from build123d import *

# Parameters (mm, degrees)
SKETCH_1_W               = 764
SKETCH_1_H               = 732
EXTRUDE_1_DEPTH          = 18
SKETCH_1_3_W             = 28
SKETCH_1_3_H             = 60
EXTRUDE_2_DEPTH          = 18
PATTERN_LINEAR_1_COUNT   = 3
PATTERN_LINEAR_1_PITCH   = 250
MIRROR_1_COPY_1_SKETCH_W = 28
MIRROR_1_COPY_1_SKETCH_H = 60
MIRROR_1_COPY_1_DEPTH    = 18
MIRROR_1_COPY_2_SKETCH_W = 28
MIRROR_1_COPY_2_SKETCH_H = 60
MIRROR_1_COPY_2_DEPTH    = 18
SKETCH_1_5_W             = 60
SKETCH_1_5_H             = 28
EXTRUDE_3_DEPTH          = 18
PATTERN_LINEAR_2_COUNT   = 3
PATTERN_LINEAR_2_PITCH   = 250
MIRROR_2_COPY_1_SKETCH_W = 60
MIRROR_2_COPY_1_SKETCH_H = 28
MIRROR_2_COPY_1_DEPTH    = 18
MIRROR_2_COPY_2_SKETCH_W = 60
MIRROR_2_COPY_2_SKETCH_H = 28
MIRROR_2_COPY_2_DEPTH    = 18
FILLET_1_R               = 25


with BuildPart() as part:
    # 草图1 → 凸台-拉伸1 (new body)
    with BuildSketch(Plane(origin=(0, 0, 0), x_dir=(1, 0, 0), z_dir=(0, 1, 0))):
        Rectangle(SKETCH_1_W, SKETCH_1_H)
    extrude(amount=EXTRUDE_1_DEPTH)

    # 草图1<3> → 凸台-拉伸2 (add)
    with BuildSketch(Plane(origin=(0, 0, 0), x_dir=(1, 0, 0), z_dir=(0, 1, 0))):
        with Locations((-396, -250)):
            Rectangle(SKETCH_1_3_W, SKETCH_1_3_H)
    extrude_2 = extrude(amount=EXTRUDE_2_DEPTH)

    # 阵列(线性)1: 凸台-拉伸2 ×3
    with Locations(*[(0, 0, -i * PATTERN_LINEAR_1_PITCH) for i in range(1, PATTERN_LINEAR_1_COUNT)]):
        add(extrude_2)

    # 镜向1: 凸台-拉伸2 across plane
    add(extrude_2.mirror(Plane(origin=(0, 0, 0), x_dir=(0, 0, 1), z_dir=(1, 0, 0))))

    # 镜向1 copy 1 sketch → 镜向1 copy 1 (add)
    with BuildSketch(Plane(origin=(0, 0, -250), x_dir=(-1, 0, 0), z_dir=(0, 1, 0))):
        with Locations((-396, 250)):
            Rectangle(MIRROR_1_COPY_1_SKETCH_W, MIRROR_1_COPY_1_SKETCH_H)
    extrude(amount=MIRROR_1_COPY_1_DEPTH)

    # 镜向1 copy 2 sketch → 镜向1 copy 2 (add)
    with BuildSketch(Plane(origin=(0, 0, -500), x_dir=(-1, 0, 0), z_dir=(0, 1, 0))):
        with Locations((-396, 250)):
            Rectangle(MIRROR_1_COPY_2_SKETCH_W, MIRROR_1_COPY_2_SKETCH_H)
    extrude(amount=MIRROR_1_COPY_2_DEPTH)

    # 草图1<5> → 凸台-拉伸3 (add)
    with BuildSketch(Plane(origin=(0, 0, 0), x_dir=(1, 0, 0), z_dir=(0, 1, 0))):
        with Locations((-250, -380)):
            Rectangle(SKETCH_1_5_W, SKETCH_1_5_H)
    extrude_3 = extrude(amount=EXTRUDE_3_DEPTH)

    # 阵列(线性)2: 凸台-拉伸3 ×3
    with Locations(*[(i * PATTERN_LINEAR_2_PITCH, 0, 0) for i in range(1, PATTERN_LINEAR_2_COUNT)]):
        add(extrude_3)

    # 镜向2: 凸台-拉伸3 across plane
    add(extrude_3.mirror(Plane.XY))

    # 镜向2 copy 1 sketch → 镜向2 copy 1 (add)
    with BuildSketch(Plane(origin=(250, 0, 0), x_dir=(1, 0, 0), z_dir=(0, 1, 0))):
        with Locations((-250, 380)):
            Rectangle(MIRROR_2_COPY_1_SKETCH_W, MIRROR_2_COPY_1_SKETCH_H)
    extrude(amount=MIRROR_2_COPY_1_DEPTH)

    # 镜向2 copy 2 sketch → 镜向2 copy 2 (add)
    with BuildSketch(Plane(origin=(500, 0, 0), x_dir=(1, 0, 0), z_dir=(0, 1, 0))):
        with Locations((-250, 380)):
            Rectangle(MIRROR_2_COPY_2_SKETCH_W, MIRROR_2_COPY_2_SKETCH_H)
    extrude(amount=MIRROR_2_COPY_2_DEPTH)

    # 圆角1
    fillet_1_edges = [part.edges().sort_by_distance(p)[0] for p in [
        (-382, 9, -366),
        (-382, 9, 366),
        (382, 9, 366),
        (382, 9, -366),
    ]]
    fillet(fillet_1_edges, radius=FILLET_1_R)


solid = part.part
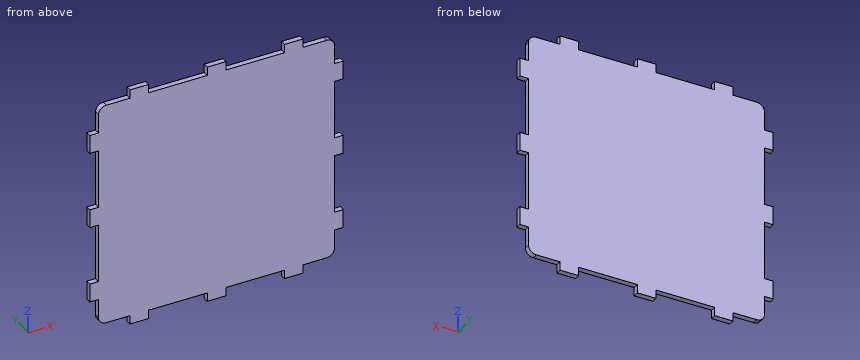
Here's how the part is built. I have some questions about the finished solid (model axes, mm). Give positions to 0.01 mm unless a question says otherwise; leave off trailing zeros. Order: outer loops, then holes, each group sorted by start corner. A loop starts at its lowest first (then second) coordinate and runs counter-clockwise, first axis right, second up. Notation, with made-up numbers: (70, 53) -> (87, 53) arc R19 ccw to (87, 88) -> close; hole circle Ø6 at (-15.5, -27.5). An arc over 180 degrees is marked (long way). Use a Markdown table: item, result. Add a question column.
Item 1: Imagine slicing it at A-A on z = 318. Please give me the cut outline in (x, y), plus the area to 3 significant figures.
Item 2: I need wall thicknesses on line 1 (Z direction, x = 69, y = 14.75); line 2 (X direction, y = 11.5, z = -35.5); line 3 (Z direction, x = 369.5, y = 1.75). Which ranges of each line are inside material? Lowest first, please.
Item 3: Will these pins go through, and if not, where does the flat tip stop? pin 1 (9 mm diameter, centred on y = 7.5, z = -318.5, fed in from -X); pin 2 (9 mm diameter, centred on y = 12.5, z = 321, fed in from +X); pin 3 (1.5 mm diameter, centred on x = 96.5, z = -5.5, fed in from -Y); pin 4 (1.5 mm diameter, centred on x = 133, y = 11, fed in from -Z).
Item 4: Imagine slicing it at B-B on x = 203.5. Please give me the cut outline in (y, z).
Data:
| question | item | result |
|---|---|---|
| 1 | outline | (-382, 0) -> (382, 0) -> (382, 18) -> (-382, 18) -> close |
| 1 | area | 13,800 mm² |
| 2 | line 1 | z = -366 to 366 |
| 2 | line 2 | x = -382 to 382 |
| 2 | line 3 | z = -362.65 to 362.65 |
| 3 | pin 1 | stops at x = -382 |
| 3 | pin 2 | stops at x = 382 |
| 3 | pin 3 | stops at y = 0 |
| 3 | pin 4 | stops at z = -366 |
| 4 | outline | (0, -366) -> (18, -366) -> (18, 366) -> (0, 366) -> close |
